Design review of the part built by this model. Coordinates are the model's own, in mm. Round coordinates to 2 decimals unless told otherwise and drop trailing zeros. Loops run counter-clockwise (first coordinate to the right, second up) from the corner with the lowest first, then second, coordinate; pieces in that order, holes last. Notation, with made-up numbers: (-29, 41) -> (15, 41) arc R4 cw to (15, 46) -> close; hole circle Ø1 at (56, 78.25). An arc over 180 degrees is marked (long way). Answer as CSV lines item,"result". Start each with the question number.
(1) Take a section at D-D, the plane x = -13.5. Write out the cut boundary in (y, z).
(2) For P1, Ø1, axis at x = 35, z = 2, coming from the +Y side; P2, Ø1, axis at y = -29.5, z = 4, coming from the +X side; P3, Ø3, axis at x = 18.5, z = 2, coming from the +Y side, all flat-tipped, find the tip position at first contact; note any pin that passes through.
(3) Take a section at B-B, the plane z = 2. Write out the cut boundary in (x, y), and give its area (3 significant figures).
(4) Take a section at C-C, the plane x = 0. Write out the cut boundary in (y, z).
(5) To check wall thickness, follow line 1 (Y direction, x = 20, z = 1.5); line 2 (X direction, y = 17.5, z = 5.5) (3 decimals); line 3 (X direction, y = -0.5, z = 5.5). State the ranges of each line that lie inside material, in increasing order. Write a range as from..to.
(6) Take a section at A-A, the plane x = 11.5. Write out the cut boundary in (y, z).
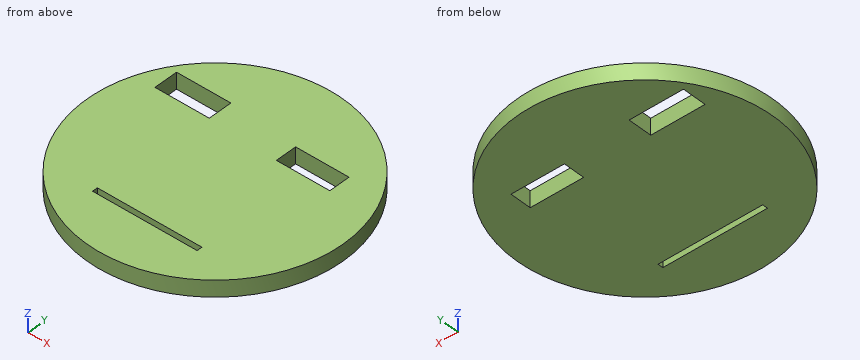
from build123d import *

# Parameters (mm, degrees)
F0_R     = 49.7916549323
F2_DEPTH = 6.35
F1_W     = 21.1281813681
F1_H     = 9.3518197536
F3_DEPTH = 6.351
F4_W     = 20.7818225026
F4_H     = 8.3127245307
F5_DEPTH = 6.351
F6_W     = 43.4686355293
F6_H     = 2.7709081769
F7_DEPTH = 145
F8_W     = 40.6977310777
F8_H     = 2.0781829953
F9_DEPTH = 6.351


# Not quite as in the source:
# - an extrude ends at something that could not be found from the text; its depth is read off the source's solid


with BuildPart() as f2:
    # F0 (on Top) → F2 (new body)
    with BuildSketch(Plane.XY):
        Circle(F0_R)
    extrude(amount=F2_DEPTH)

    # F1 (on face) → F3 (cut, through all)
    with BuildSketch(Plane.XY):
        with Locations((-28.1420461833, 21.7343177646)):
            Rectangle(F1_W, F1_H)
    extrude(amount=F3_DEPTH, mode=Mode.SUBTRACT)

    # F4 (on Top) → F5 (cut, through all)
    with BuildSketch(Plane.XY):
        with Locations((20.1756805182, 19.8293179274)):
            Rectangle(F4_W, F4_H)
    extrude(amount=F5_DEPTH, mode=Mode.SUBTRACT)

    # F6 (on face) → F7 (cut, through all)
    with BuildSketch(Plane.XY.offset(6.35)):
        with Locations((0, -21.9075009227)):
            Rectangle(F6_W, F6_H)
    extrude(amount=F7_DEPTH, mode=Mode.SUBTRACT)

    # F8 (on Top) → F9 (cut, through all)
    with BuildSketch(Plane.XY):
        with Locations((0, -29.3543189764)):
            Rectangle(F8_W, F8_H)
    extrude(amount=F9_DEPTH, mode=Mode.SUBTRACT)


solid = f2.part
The answers:
1,outline,"(-47.93, 0) -> (-30.39, 0) -> (-30.39, 6.35) -> (-47.93, 6.35) -> close; (-28.32, 0) -> (47.93, 0) -> (47.93, 6.35) -> (-28.32, 6.35) -> close"
2,P1,"y = 35.9"
2,P2,"x = 40.47"
2,P3,"y = 46.8"
3,outline,"circle Ø99.58 at (0, 0); hole (-38.71, 17.06) -> (-17.58, 17.06) -> (-17.58, 26.41) -> (-38.71, 26.41) -> close; hole (-20.35, -30.39) -> (20.35, -30.39) -> (20.35, -28.32) -> (-20.35, -28.32) -> close; hole (9.78, 15.67) -> (30.57, 15.67) -> (30.57, 23.99) -> (9.78, 23.99) -> close"
3,area,"7,330 mm²"
4,outline,"(-49.79, 0) -> (-30.39, 0) -> (-30.39, 6.35) -> (-49.79, 6.35) -> close; (-28.32, 0) -> (49.79, 0) -> (49.79, 6.35) -> (-28.32, 6.35) -> close"
5,line 1,"-45.6..-30.39, -28.32..15.67, 23.99..45.6"
5,line 2,"-46.615..-38.706, -17.578..9.785, 30.567..46.615"
5,line 3,"-49.79..49.79"
6,outline,"(-48.45, 0) -> (-30.39, 0) -> (-30.39, 6.35) -> (-48.45, 6.35) -> close; (-28.32, 0) -> (15.67, 0) -> (15.67, 6.35) -> (-28.32, 6.35) -> close; (23.99, 0) -> (48.45, 0) -> (48.45, 6.35) -> (23.99, 6.35) -> close"
